```python
from build123d import *

# Parameters (mm, degrees)
SKIZZE1_R                         = 2.15
AUFSATZ_LINEAR_AUSTRAGEN1_DEPTH   = 12
AUFSATZ_LINEAR_AUSTRAGEN1_2_DEPTH = 12
AUFSATZ_LINEAR_START              = 7
SKIZZE1_3_W                       = 10
SKIZZE1_3_H                       = 34
SKIZZE1_3_R                       = 2.15
SKIZZE1_3_R_2                     = 2.5
AUFSATZ_LINEAR_AUSTRAGEN3_DEPTH   = 7
SKIZZE4_W                         = 52.5
SKIZZE4_H                         = 72.5
SKIZZE4_R                         = 2.5
SKIZZE4_R_2                       = 2.15
AUFSATZ_LINEAR_AUSTRAGEN4_DEPTH   = 7
SKIZZE4_3_R                       = 2.5
SKIZZE4_3_R_2                     = 1.25
AUFSATZ_LINEAR_AUSTRAGEN5_DEPTH   = 2.5
SCHNITT_LINEAR_START              = -7
SKIZZE4_4_R                       = 1.25
SCHNITT_LINEAR_AUSTRAGEN1_DEPTH   = 7
SKIZZE4_5_R                       = 2.15
SCHNITT_LINEAR_AUSTRAGEN2_DEPTH   = 19
SKIZZE6_W                         = 62.5
SKIZZE6_H                         = 82.5
SKIZZE6_W_2                       = 52.5
SKIZZE6_H_2                       = 72.5
AUFSATZ_LINEAR_AUSTRAGEN6_DEPTH   = 7
SKIZZE5_R                         = 1.25
SCHNITT_LINEAR_AUSTRAGEN3_DEPTH   = 7


with BuildPart() as part:
    # Skizze1 → Aufsatz-Linear austragen1 (new body)
    with BuildSketch(Plane.XY):
        with Locations((-14.25, 0)):
            Circle(SKIZZE1_R)
    extrude(amount=-AUFSATZ_LINEAR_AUSTRAGEN1_DEPTH)



with BuildPart() as body_2:
    # Skizze1 → Aufsatz-Linear austragen1 2 (new body)
    with BuildSketch(Plane.XY):
        with Locations((14.25, 0)):
            Circle(SKIZZE1_R)
    extrude(amount=-AUFSATZ_LINEAR_AUSTRAGEN1_2_DEPTH)


with BuildPart() as part_1:
    add(part.part)

    add(body_2.part)  # Aufsatz-Linear austragen3 merges body 2
    # Skizze1<3> → Aufsatz-Linear austragen3 (add)
    # profile 1 of 4: a face of its own
    with BuildSketch(Plane.XY.offset(AUFSATZ_LINEAR_START)):
        with Locations((-12.5, 0)):
            Rectangle(SKIZZE1_3_W, SKIZZE1_3_H)
        with Locations((-14.25, 0)):
            Circle(SKIZZE1_3_R, mode=Mode.SUBTRACT)
    # profile 2 of 4: a face of its own
    with BuildSketch(Plane.XY.offset(AUFSATZ_LINEAR_START)):
        Polygon((17.5, -17), (17.5, 17), (0, 17), (-7.5, 17), (-7.5, -17), align=None)
        with Locations((0, -7)):
            Circle(SKIZZE1_3_R_2, mode=Mode.SUBTRACT)
        with Locations((0, 7)):
            Circle(SKIZZE1_3_R_2, mode=Mode.SUBTRACT)
        with Locations((14.25, 0)):
            Circle(SKIZZE1_3_R, mode=Mode.SUBTRACT)
    # profile 3 of 4: a face of its own
    with BuildSketch(Plane.XY.offset(AUFSATZ_LINEAR_START)):
        with Locations((-14.25, 0)):
            Circle(SKIZZE1_3_R)
    # profile 4 of 4: a face of its own
    with BuildSketch(Plane.XY.offset(AUFSATZ_LINEAR_START)):
        with Locations((14.25, 0)):
            Circle(SKIZZE1_3_R)
    extrude(amount=-AUFSATZ_LINEAR_AUSTRAGEN3_DEPTH)

    # Skizze4 → Aufsatz-Linear austragen4 (add)
    with BuildSketch(Plane.XY.offset(7)):
        with Locations((1.25, -6.25)):
            Rectangle(SKIZZE4_W, SKIZZE4_H)
        with Locations((0, -7)):
            Circle(SKIZZE4_R, mode=Mode.SUBTRACT)
        with Locations((-14.25, 0)):
            Circle(SKIZZE4_R_2, mode=Mode.SUBTRACT)
        with Locations((0, 7)):
            Circle(SKIZZE4_R, mode=Mode.SUBTRACT)
        with Locations((14.25, 0)):
            Circle(SKIZZE4_R_2, mode=Mode.SUBTRACT)
    extrude(amount=-AUFSATZ_LINEAR_AUSTRAGEN4_DEPTH)

    # Skizze4<3> → Aufsatz-Linear austragen5 (add)
    # profile 1 of 4: a face of its own
    with BuildSketch(Plane.XY.offset(7)):
        with Locations((-12.5, -20)):
            Circle(SKIZZE4_3_R)
        with Locations((-12.5, -20)):
            Circle(SKIZZE4_3_R_2, mode=Mode.SUBTRACT)
    # profile 2 of 4: a face of its own
    with BuildSketch(Plane.XY.offset(7)):
        with Locations((-12.5, 20)):
            Circle(SKIZZE4_3_R)
        with Locations((-12.5, 20)):
            Circle(SKIZZE4_3_R_2, mode=Mode.SUBTRACT)
    # profile 3 of 4: a face of its own
    with BuildSketch(Plane.XY.offset(7)):
        with Locations((20, 20)):
            Circle(SKIZZE4_3_R)
        with Locations((20, 20)):
            Circle(SKIZZE4_3_R_2, mode=Mode.SUBTRACT)
    # profile 4 of 4: a face of its own
    with BuildSketch(Plane.XY.offset(7)):
        with Locations((20, -20)):
            Circle(SKIZZE4_3_R)
        with Locations((20, -20)):
            Circle(SKIZZE4_3_R_2, mode=Mode.SUBTRACT)
    extrude(amount=AUFSATZ_LINEAR_AUSTRAGEN5_DEPTH)

    # Skizze4<4> → Schnitt-Linear austragen1 (cut)
    with BuildSketch(Plane.XY.offset(7).offset(SCHNITT_LINEAR_START)):
        with Locations((-12.5, -20)):
            Circle(SKIZZE4_4_R)
        with Locations((20, 20)):
            Circle(SKIZZE4_4_R)
        with Locations((20, -20)):
            Circle(SKIZZE4_4_R)
        with Locations((-12.5, 20)):
            Circle(SKIZZE4_4_R)
    extrude(amount=SCHNITT_LINEAR_AUSTRAGEN1_DEPTH, mode=Mode.SUBTRACT)

    # Skizze4<5> → Schnitt-Linear austragen2 (cut)
    with BuildSketch(Plane.XY.offset(7)):
        with Locations((-14.25, 0)):
            Circle(SKIZZE4_5_R)
        with Locations((14.25, 0)):
            Circle(SKIZZE4_5_R)
    extrude(amount=-SCHNITT_LINEAR_AUSTRAGEN2_DEPTH, mode=Mode.SUBTRACT)

    # Skizze6 → Aufsatz-Linear austragen6 (add)
    with BuildSketch(Plane.XY.offset(7)):
        with Locations((1.25, -6.25)):
            Rectangle(SKIZZE6_W, SKIZZE6_H)
        with Locations((1.25, -6.25)):
            Rectangle(SKIZZE6_W_2, SKIZZE6_H_2, mode=Mode.SUBTRACT)
    extrude(amount=-AUFSATZ_LINEAR_AUSTRAGEN6_DEPTH)

    # Skizze5 → Schnitt-Linear austragen3 (cut)
    with BuildSketch(Plane.XY.offset(7)):
        with Locations((-27.5, 32.5)):
            Circle(SKIZZE5_R)
        with Locations((-27.5, -45)):
            Circle(SKIZZE5_R)
        with Locations((30, -45)):
            Circle(SKIZZE5_R)
        with Locations((30, 32.5)):
            Circle(SKIZZE5_R)
    extrude(amount=-SCHNITT_LINEAR_AUSTRAGEN3_DEPTH, mode=Mode.SUBTRACT)


solid = part_1.part
```
Design review of the part built by this model. Coordinates are the model's own, in mm. A direction names the side the tool comes from. Round coordinates to 2 decimals unless told otherwise and drop trailing zeros. Write each loop counter-clockwise with the first axis right and the second up, starting at its lowest first coordinate (ties: lowest second). Pieces come first, ordered by that corner, then holes.
Item 1: The part is to be moulded in two halves that separate along Y. For faces 1 (the flat face through (19, 19, 9.5)), 2 (the cylindrical face through (-12.2, 0.65, 3.55)), say which applies: +Y half, -Y half, draft (parallel to the pull), parting line (faces both ways), or undercut.
Item 2: We need section C-C on x = -27.5. Write out the cut boundary in (y, z), and give its area (4 significant figures).
Item 3: We need section B-B on z = 8.25. Write out the cut boundary in (x, y).
Item 4: For probe 1 along Y at (x, z) = (0, 5.5); probe 2 along Y at (x, z) = (-1.5, 1.25); probe 3 along X at (y, z) = (-20.5, 2.25), list the stretches that pass through material, from the lowest coordinate up.
Item 5: Clearance check with flat-ended pins moving along their axes: pin 1 Ø8 at (x, y) = (19.5, 17.5) entering from +Z; pin 2 Ø2 at (x, y) = (20, 20) entering from -Z; pin 3 Ø1 at (x, y) = (24, 24.5) entering from +Z. State where each tip first meets the part, or that it passes through.
Item 6: We need section D-D on y = -5.5. Write out the cut boundary in (x, z), and give its area (4 significant figures).
Item 7: For faces 3 (the cylindrical face through (31.155, 32.021, 3.549)), 4 (the cylindrical face through (-14, -18, 8)), list the 3-axis set-ups (+Z, -Z, +X, -X, +Y, -Y) from which the entire face can be reached by the end or side of a thin tool; tool diameter is ignored.
Item 8: We need section A-A on y = -20. Write out the cut boundary in (x, z).
Returned:
1. face 1: draft
1. face 2: undercut
2. outline: (-47.5, 0) - (-46.25, 0) - (-46.25, 7) - (-47.5, 7) - close; (-43.75, 0) - (31.25, 0) - (31.25, 7) - (-43.75, 7) - close; (33.75, 0) - (35, 0) - (35, 7) - (33.75, 7) - close
2. area: 542.5 mm2
3. outline: circle Ø5 at (-12.5, -20); circle Ø5 at (-12.5, 20); circle Ø5 at (20, -20); circle Ø5 at (20, 20); hole circle Ø2.5 at (-12.5, -20); hole circle Ø2.5 at (-12.5, 20); hole circle Ø2.5 at (20, -20); hole circle Ø2.5 at (20, 20)
4. probe 1: y = -47.5 to -9.5, -4.5 to 4.5, 9.5 to 35
4. probe 2: y = -47.5 to -9, -5 to 5, 9 to 35
4. probe 3: x = -30 to -13.65, -11.35 to 18.85, 21.15 to 32.5
5. pin 1: stops at z = 9.5
5. pin 2: passes through
5. pin 3: stops at z = 7
6. outline: (-30, 0) - (-2, 0) - (-2, 7) - (-30, 7) - close; (2, 0) - (32.5, 0) - (32.5, 7) - (2, 7) - close
6. area: 409.5 mm2
7. face 3: +Z, -Z
7. face 4: +Z
8. outline: (-30, 0) - (-13.75, 0) - (-13.75, 9.5) - (-15, 9.5) - (-15, 7) - (-30, 7) - close; (-11.25, 0) - (18.75, 0) - (18.75, 9.5) - (17.5, 9.5) - (17.5, 7) - (-10, 7) - (-10, 9.5) - (-11.25, 9.5) - close; (21.25, 0) - (32.5, 0) - (32.5, 7) - (22.5, 7) - (22.5, 9.5) - (21.25, 9.5) - close
